Part print with two shaded views. Sizes in mm from the minimum x, y, z corner. A direction names the side the tool comes from. Round coordinates to 2 decimals unless told otherwise and drop trailing zeros. Write each loop counter-clockwise with the first axis right and the second up, starting at its lowest first coordinate (ties: lowest second). Pieces come first, ordered by that corner, then holes. Notation, with made-up numbers: (-17, 27) - (23, 27) arc R33 ccw to (23, 58) - close; hole circle Ø11 at (7.25, 37.25). An arc over 180 degrees is marked (long way). Answer as a JSON object with one key per item and string values. Group by question number.
Item 1: Slice it at B-B, the plane z = 11.5. List the corners of the cut face in (x, y) (3 decimals).
Item 2: Probe line 1 (X direction, y = 69, z = 11) (1 decimal); line 2 (Z direction, x = 12, y = 68) (1 decimal); line 3 (Y direction, x = 25.5, z = 35.5). List the from-to ranges inside material, lowest first. Write a range as from..to.
Item 3: Slice it at D-D, the plane x = 52.8. List the corners of the cut face in (y, z) (3 decimals).
Item 4: Which spindle directions (+Z, -Z, +X, -X, +Y, -Y) get a long thin tool onto all of the face, cutting with end or side? Do the marked faces 1 and 2. Say none if no direction does.
Item 5: Slice it at C-C, the plane x = 29.5. List the corners of the cut face in (y, z) (3 decimals), then the cut area to 3 significant figures.
Item 6: Slice it at A-A, the plane x = 38. List the corners of the cut face in (y, z).
Item 7: Flat gauge pins, fed straight in: pin 1 (2.5 mm diameter, centred on x = 29.5, z = 5, fed in from -Y); pin 2 (5.5 mm diameter, centred on x = 16.5, y = 69, fed in from -Z); pin 3 (1 mm diameter, centred on y = 45, z = 25, fed in from +X); pin 4 (1 mm diameter, centred on x = 1.5, y = 13.5, fed in from -Z). Where does each tip first touch, or does it go through?
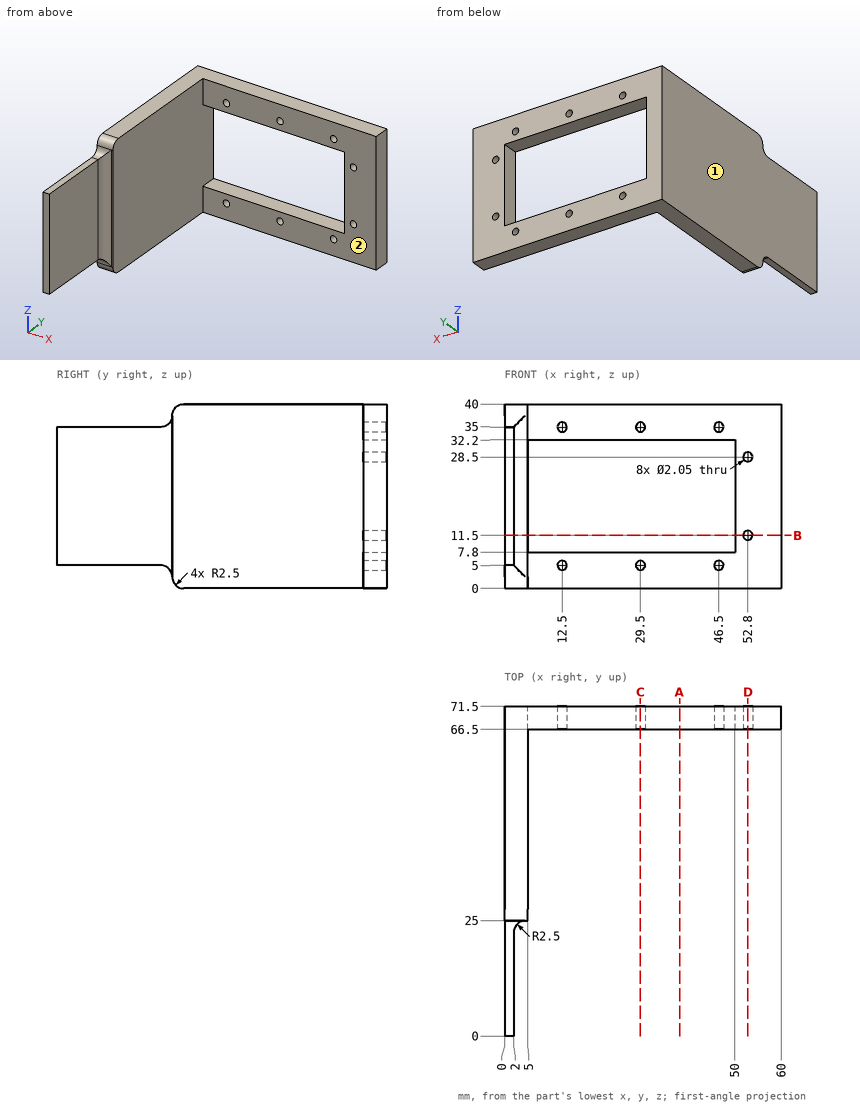
Geometry says:
{
 "1": {"outline": "(0, 0) - (2, 0) - (2, 22.5) arc R2.5 cw to (4.5, 25) - (5, 25) - (5, 71.5) - (0, 71.5) - close; (50, 66.5) - (51.775, 66.5) - (51.775, 71.5) - (50, 71.5) - close; (53.825, 66.5) - (60, 66.5) - (60, 71.5) - (53.825, 71.5) - close"},
 "2": {"line 1": "x = 0..5, 50..51.9, 53.7..60", "line 2": "z = 0..4.1, 5.9..7.8, 32.2..34.1, 35.9..40", "line 3": "y = 66.5..71.5"},
 "3": {"outline": "(66.5, 0) - (71.5, 0) - (71.5, 10.475) - (66.5, 10.475) - close; (66.5, 12.525) - (71.5, 12.525) - (71.5, 27.475) - (66.5, 27.475) - close; (66.5, 29.525) - (71.5, 29.525) - (71.5, 40) - (66.5, 40) - close"},
 "4": {"face 1": "+Z, -Z, -X, +Y, -Y", "face 2": "+Z, -Z, +X, -Y"},
 "5": {"outline": "(66.5, 0) - (71.5, 0) - (71.5, 3.975) - (66.5, 3.975) - close; (66.5, 6.025) - (71.5, 6.025) - (71.5, 7.8) - (66.5, 7.8) - close; (66.5, 32.2) - (71.5, 32.2) - (71.5, 33.975) - (66.5, 33.975) - close; (66.5, 36.025) - (71.5, 36.025) - (71.5, 40) - (66.5, 40) - close", "area": "57.5 mm^2"},
 "6": {"outline": "(66.5, 0) - (71.5, 0) - (71.5, 7.8) - (66.5, 7.8) - close; (66.5, 32.2) - (71.5, 32.2) - (71.5, 40) - (66.5, 40) - close"},
 "7": {"pin 1": "stops at y = 66.5", "pin 2": "stops at z = 0", "pin 3": "stops at x = 5", "pin 4": "stops at z = 5"}
}
